Source: CAD feature listing. Evaluate the final solid. Frame: model axes, mm. A direction names the side the tool comes from. Give positions to 0.01 mm unless a question says otherwise; leave off trailing zeros. Loops run counter-clockwise (first coordinate to the right, second up) from the corner with the lowest first, then second, coordinate; pieces in that order, holes last. Notation, with made-up numbers: M 46,-7 L 63,-7 A16 ccw 63,-3 Z; hole C 22,-8 d4. An arc over 180 degrees is marked long. Answer in a Markdown table with one row per item.
```python
from build123d import *

# Parameters (mm, degrees)
ESBO_O1_R                = 15
ESBO_O1_R_2              = 1
RESSALTO_EXTRUS_O1_DEPTH = 10
ESBO_O2_R                = 10.25
ESBO_O2_R_2              = 3.75
CORTE_EXTRUS_O1_DEPTH    = 4


with BuildPart() as part:
    # Esboço1 → Ressalto-extrusão1 (new body)
    with BuildSketch(Plane.XY):
        Circle(ESBO_O1_R)
        Circle(ESBO_O1_R_2, mode=Mode.SUBTRACT)
    extrude(amount=RESSALTO_EXTRUS_O1_DEPTH)

    # Esboço2 → Corte-extrusão1 (cut)
    with BuildSketch(Plane.XY.offset(10)):
        Circle(ESBO_O2_R)
        Circle(ESBO_O2_R_2, mode=Mode.SUBTRACT)
    extrude(amount=-CORTE_EXTRUS_O1_DEPTH, mode=Mode.SUBTRACT)


solid = part.part
```
1) Pin query (flat end, axial travel): pin 1 Ø1 at (y, z) = (-7.5, 4.5) entering from -X; pin 2 Ø1.5 at (x, y) = (-6, 4) entering from +Z; pin 3 Ø1.8 at (x, y) = (0, 0) entering from +Z; pin 4 Ø1.5 at (x, z) = (6.5, 6.5) entering from +Y. Return the tip coordinate at first contact, or that it passes through.
Reply:
| item | result |
|---|---|
| pin 1 | stops at x = -13.27 |
| pin 2 | stops at z = 6 |
| pin 3 | passes through |
| pin 4 | stops at y = 13.85 |
2) Set-up query: faces 1 (the flat face through (1, -1, 10)), 2 (the flat face through (4, 0, 6)). Return all of +Z, -Z, +X, -X, +Y, -Y with unobstructed straight access to the full face (end or side cutting, diameter ignored); none if empty.
Reply:
| item | result |
|---|---|
| face 1 | +Z, +X, -X, +Y, -Y |
| face 2 | +Z |
3) Section A-A, the plane y = 0. Return loops of the section in (x, z), then the cut area to 3 significant figures.
Reply:
| item | result |
|---|---|
| outline | M -15,0 L -1,0 L -1,10 L -3.75,10 L -3.75,6 L -10.25,6 L -10.25,10 L -15,10 Z; M 1,0 L 15,0 L 15,10 L 10.25,10 L 10.25,6 L 3.75,6 L 3.75,10 L 1,10 Z |
| area | 228 mm² |
4) Pull-direction query (X, two-part tool) for faces 3 (the cylindrical face through (-14.985, 0.66, 4.93)), 4 (the cylindrical face through (-2.222, -10.006, 8.028)), 5 (the flat face through (3, 0, 0)), 6 (the cylindrical face through (0, -1, 5)); classes: released by +X, released by -X, zero draft, split by the parting line, or undercut.
Reply:
| item | result |
|---|---|
| face 3 | split by the parting line |
| face 4 | undercut |
| face 5 | zero draft |
| face 6 | undercut |
5) Section C-C, the plane x = 7.25. Return loops of the section in (y, z), then the cut area to 3 significant figures.
Reply:
| item | result |
|---|---|
| outline | M -13.13,0 L 13.13,0 L 13.13,10 L 7.25,10 L 7.25,6 L -7.25,6 L -7.25,10 L -13.13,10 Z |
| area | 205 mm² |
6) Material intervals for L1, parallel to Y at x = 0, z = 7; L2, parallel to X at y = 3, z = 7.75; L3, parallel to Y at x = 0, z = 3.5, sorted ascending.
Reply:
| item | result |
|---|---|
| L1 | y = -15 to -10.25, -3.75 to -1, 1 to 3.75, 10.25 to 15 |
| L2 | x = -14.7 to -9.8, -2.25 to 2.25, 9.8 to 14.7 |
| L3 | y = -15 to -1, 1 to 15 |
7) Section D-D, the plane z = 2.25. Return loops of the section in (x, y).
Reply:
| item | result |
|---|---|
| outline | C 0,0 d30; hole C 0,0 d2 |
